Model file for the job. Use its own axes, mm. A direction names the side the tool comes from. Give positions to 0.01 mm unless a question says otherwise; leave off trailing zeros. Return JSON: item names as keys, results as strings. Group by question number.
1. Two-plate mould, pull along X, no slides. Class faces 1 (the face through (26, 0, 1)), 2 (the face through (-31, 8, 1)), 3 (the face through (-34, -2, 1)): released by +X, released by -X, zero draft, split by the parting line, or undercut.
2. Wall check: probe 1 along X at (y, z) = (5.5, 2.45); probe 2 along X at (y, z) = (1.5, 2.8); probe 3 along Y at (x, z) = (-28.5, 2.15). Give the ranges that are in metal, low to high. Write a range as [from, to].
3. Pin check, flat tips, straight feed: pin 1 (3 mm diameter, centred on x = 0, y = -31, fed in from +Z); pin 2 (0.9 mm diameter, centred on x = -29.5, z = 1.5, fed in from +Y); pin 3 (1 mm diameter, centred on x = -3, z = 1.5, fed in from -Y). Stop position of each tip, or through.
4. Slice it at A-A on z = 0.8. Give the number of separate pieces and of enclosed holes in the cut face, then the cut area to 3 significant figures.
5. 3-axis set-ups, long thin cutter, end or side, ignore diameter. For faces 4 (the face through (-30, -12, 1)), 5 (the face through (0, 29, 1)): which of +Z, -Z, +X, -X, +Y, -Y reach the whole face in a straight line?
from build123d import *

# Parameters (mm, degrees)
ESQUISSE1_RX            = 35
ESQUISSE1_RY            = 28
ESQUISSE1_R             = 2
BOSS_EXTRU_1_DEPTH      = 3
ESQUISSE2_R             = 2
ENL_V_MAT_EXTRU_1_DEPTH = 10
ESQUISSE4_W             = 8
ESQUISSE4_H             = 20
BOSS_EXTRU_2_DEPTH      = 3
ESQUISSE3_R             = 1.5
ENL_V_MAT_EXTRU_2_DEPTH = 10


with BuildPart() as part:
    # Esquisse1 → Boss.-Extru.1 (new body)
    with BuildSketch(Plane.XY):
        with Locations(Location((0, 0), (0, 0, 90))):
            Ellipse(ESQUISSE1_RX, ESQUISSE1_RY)
        with Locations((0, 20)):
            Circle(ESQUISSE1_R, mode=Mode.SUBTRACT)
        with Locations((0, -20)):
            Circle(ESQUISSE1_R, mode=Mode.SUBTRACT)
    extrude(amount=BOSS_EXTRU_1_DEPTH)

    # Esquisse2 → Enlèv. mat.-Extru.1 (cut)
    with BuildSketch(Plane(origin=(0, 0, 0), x_dir=(-1, 0, 0), z_dir=(0, 0, -1))):
        with Locations((24, 0)):
            Circle(ESQUISSE2_R)
        with Locations((-24, 0)):
            Circle(ESQUISSE2_R)
        with Locations((0, 31)):
            Circle(ESQUISSE2_R)
        with Locations((0, -31)):
            Circle(ESQUISSE2_R)
    extrude(amount=-ENL_V_MAT_EXTRU_1_DEPTH, mode=Mode.SUBTRACT)

    # Esquisse4 → Boss.-Extru.2 (add)
    with BuildSketch(Plane(origin=(0, 0, 0), x_dir=(-1, 0, 0), z_dir=(0, 0, -1))):
        with Locations((30, -2)):
            Rectangle(ESQUISSE4_W, ESQUISSE4_H)
    extrude(amount=-BOSS_EXTRU_2_DEPTH)

    # Esquisse3 → Enlèv. mat.-Extru.2 (cut)
    with BuildSketch(Plane(origin=(0, 0, 0), x_dir=(-1, 0, 0), z_dir=(0, 0, -1))):
        with Locations((5, 5)):
            Circle(ESQUISSE3_R)
        with Locations((31, 5)):
            Circle(ESQUISSE3_R)
    extrude(amount=-ENL_V_MAT_EXTRU_2_DEPTH, mode=Mode.SUBTRACT)


solid = part.part
Result:
{
 "1": {"face 1": "undercut", "face 2": "zero draft", "face 3": "released by -X"},
 "2": {"probe 1": "x = [-34, -32.41], [-29.59, -6.41], [-3.59, 27.65]", "probe 2": "x = [-34, -25.32], [-22.68, 22.68], [25.32, 27.97]", "probe 3": "y = [-12, 8]"},
 "3": {"pin 1": "passes through", "pin 2": "stops at y = 8", "pin 3": "stops at y = -34.86"},
 "4": {"separate pieces": "1", "enclosed holes": "8", "area": "3,120 mm2"},
 "5": {"face 4": "+Z, -Z, -X, -Y", "face 5": "+Z, -Z"}
}
